Build history of the part. All positions in model axes, mm. Face numbers are marked on the shaded views. A direction names the side the tool comes from. Coordinates: 2 decimals unless noted, no trailing zeros. Write each loop counter-clockwise with the first axis right and the second up, starting at its lowest first coordinate (ties: lowest second). Pieces come first, ordered by that corner, then holes. Notation, with made-up numbers: M 40.25,83.25 L 50.25,83.25 A18 cw 50.25,115.25 Z; hole C -3.75,75.5 d8. An arc over 180 degrees is marked long. Use CSV: the item, a comma, the result in double quotes. Start each with the question number.
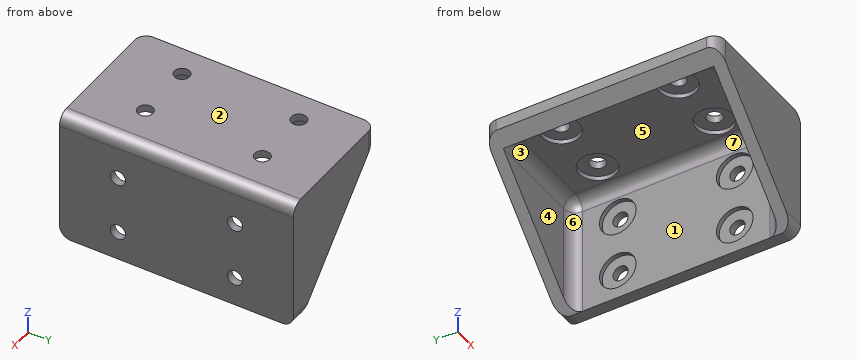
```python
from build123d import *

# Parameters (mm, degrees)
SKETCH1_W           = 45
SKETCH1_H           = 80
BOSS_EXTRUDE1_DEPTH = 45
SKETCH3_R           = 2.6
CUT_EXTRUDE1_DEPTH  = 40
SHELL1_OUTLINE_R    = 6.6
SHELL1_DEPTH        = 41
SHELL1_2_OUTLINE_R  = 6.6
SHELL1_2_DEPTH      = 1
CUT_EXTRUDE2_DEPTH  = 96.338073399
SKETCH5_W           = 37
SKETCH5_H           = 72
CUT_EXTRUDE3_DEPTH  = 40
SKETCH6_R           = 2.6
CUT_EXTRUDE4_DEPTH  = 40
FILLET1_R           = 4
FILLET2_R           = 4
FILLET3_R           = 4
SKETCH8_R           = 6.25
CUT_EXTRUDE5_DEPTH  = 1.5
SKETCH7_R           = 6.25
CUT_EXTRUDE6_DEPTH  = 1.5


# Read off the part's stored shape, not the designer's step: Shell1
with BuildPart() as part:
    # Sketch1 → Boss-Extrude1 (new body)
    with BuildSketch(Plane.XY):
        with Locations((3.274953722, 5.904112676)):
            Rectangle(SKETCH1_W, SKETCH1_H)
    extrude(amount=BOSS_EXTRUDE1_DEPTH)

    # Sketch3 → Cut-Extrude1 (cut)
    with BuildSketch(Plane(origin=(0, 0, 45), x_dir=(-1, 0, 0), z_dir=(0, 0, 1))):
        with Locations(Location((-10.774953722, -25.904112676, 0), (0, 0, 180))):
            Circle(SKETCH3_R)
        with Locations(Location((-10.774953722, 14.095887324, 0), (0, 0, 180))):
            Circle(SKETCH3_R)
        with Locations(Location((9.225046278, 14.095887324, 0), (0, 0, 180))):
            Circle(SKETCH3_R)
        with Locations(Location((9.225046278, -25.904112676, 0), (0, 0, 180))):
            Circle(SKETCH3_R)
    extrude(amount=-CUT_EXTRUDE1_DEPTH, mode=Mode.SUBTRACT)

    # Shell1 outline → Shell1 (cut)
    with BuildSketch(Plane.XY):
        with BuildLine():
            Line((-15.225046278, -16.845432741), (-15.225046278, -30.095887324))
            Line((-15.225046278, -30.095887324), (21.774953722, -30.095887324))
            Line((21.774953722, -30.095887324), (21.774953722, 41.904112676))
            Line((21.774953722, 41.904112676), (-15.225046278, 41.904112676))
            Line((-15.225046278, 41.904112676), (-15.225046278, 28.653658093))
            ThreePointArc((-15.225046278, 28.653658093), (-2.625046278, 25.904112676), (-15.225046278, 23.154567259))
            Line((-15.225046278, 23.154567259), (-15.225046278, -11.346341907))
            ThreePointArc((-15.225046278, -11.346341907), (-2.625046278, -14.095887324), (-15.225046278, -16.845432741))
        make_face()
        with Locations((10.774953722, -14.095887324)):
            Circle(SHELL1_OUTLINE_R, mode=Mode.SUBTRACT)
        with Locations((10.774953722, 25.904112676)):
            Circle(SHELL1_OUTLINE_R, mode=Mode.SUBTRACT)
    extrude(amount=SHELL1_DEPTH, mode=Mode.SUBTRACT)

    # Shell1 2 outline → Shell1 2 (cut)
    with BuildSketch(Plane.XY):
        with BuildLine():
            Line((-15.225046278, -11.346341907), (-15.225046278, -16.845432741))
            ThreePointArc((-15.225046278, -16.845432741), (-2.625046278, -14.095887324), (-15.225046278, -11.346341907))
        make_face()
        with BuildLine():
            Line((-15.225046278, 28.653658093), (-15.225046278, 23.154567259))
            ThreePointArc((-15.225046278, 23.154567259), (-2.625046278, 25.904112676), (-15.225046278, 28.653658093))
        make_face()
        with Locations((10.774953722, -14.095887324)):
            Circle(SHELL1_2_OUTLINE_R)
        with Locations((10.774953722, 25.904112676)):
            Circle(SHELL1_2_OUTLINE_R)
    extrude(amount=SHELL1_2_DEPTH, mode=Mode.SUBTRACT)

    # Sketch4 → Cut-Extrude2 (cut, through all)
    with BuildSketch(Plane(origin=(0, 45.904112676, 0), x_dir=(1, 0, 0), z_dir=(0, 1, 0))):
        Polygon((-19.225046278, 0), (-19.225046278, -41), (21.774953722, 0), align=None)
    extrude(amount=-CUT_EXTRUDE2_DEPTH, mode=Mode.SUBTRACT)

    # Sketch5 → Cut-Extrude3 (cut)
    with BuildSketch(Plane(origin=(0, 0, 41), x_dir=(-1, 0, 0), z_dir=(0, 0, -1))):
        with Locations((-3.274953722, 5.904112676)):
            Rectangle(SKETCH5_W, SKETCH5_H)
    extrude(amount=CUT_EXTRUDE3_DEPTH, mode=Mode.SUBTRACT)

    # Sketch6 → Cut-Extrude4 (cut)
    with BuildSketch(Plane(origin=(25.774953722, 0, 0), x_dir=(0, 0, 1), z_dir=(1, 0, 0))):
        with Locations(Location((10, -25.904112676, 0), (0, 0, 180))):
            Circle(SKETCH6_R)
        with Locations(Location((10, 14.095887324, 0), (0, 0, 180))):
            Circle(SKETCH6_R)
        with Locations(Location((30, 14.095887324, 0), (0, 0, 180))):
            Circle(SKETCH6_R)
        with Locations(Location((30, -25.904112676, 0), (0, 0, 180))):
            Circle(SKETCH6_R)
    extrude(amount=-CUT_EXTRUDE4_DEPTH, mode=Mode.SUBTRACT)

    # Fillet1
    fillet1_edges = [part.edges().sort_by_distance(p)[0] for p in [
        (3.274953722, -30.095887324, 41),
        (21.774953722, -30.095887324, 20.5),
        (21.774953722, 41.904112676, 20.5),
        (21.774953722, 5.904112676, 41),
        (3.274953722, 41.904112676, 41),
    ]]
    fillet(fillet1_edges, radius=FILLET1_R)

    # Fillet2
    fillet2_edges = [part.edges().sort_by_distance(p)[0] for p in [
        (23.774953722, -34.095887324, 0),
        (23.774953722, 45.904112676, 0),
        (-19.225046278, -34.095887324, 43),
        (-19.225046278, 45.904112676, 43),
    ]]
    fillet(fillet2_edges, radius=FILLET2_R)

    # Fillet3
    fillet3_edges = [part.edges().sort_by_distance(p)[0] for p in [
        (25.774953722, 5.904112676, 45),
    ]]
    fillet(fillet3_edges, radius=FILLET3_R)

    # Sketch8 → Cut-Extrude5 (cut)
    with BuildSketch(Plane(origin=(0, 0, 41), x_dir=(-1, 0, 0), z_dir=(0, 0, -1))):
        with Locations((-10.774953722, -14.095887324)):
            Circle(SKETCH8_R)
        with Locations((-10.774953722, 25.904112676)):
            Circle(SKETCH8_R)
        with Locations((9.225046278, 25.904112676)):
            Circle(SKETCH8_R)
        with Locations((9.225046278, -14.095887324)):
            Circle(SKETCH8_R)
    extrude(amount=-CUT_EXTRUDE5_DEPTH, mode=Mode.SUBTRACT)

    # Sketch7 → Cut-Extrude6 (cut)
    with BuildSketch(Plane.ZY.offset(-21.774953722)):
        with Locations((10, 25.904112676)):
            Circle(SKETCH7_R)
        with Locations((30, 25.904112676)):
            Circle(SKETCH7_R)
        with Locations((30, -14.095887324)):
            Circle(SKETCH7_R)
        with Locations((10, -14.095887324)):
            Circle(SKETCH7_R)
    extrude(amount=-CUT_EXTRUDE6_DEPTH, mode=Mode.SUBTRACT)


solid = part.part
```
1. 3-axis set-ups, long thin cutter, end or side, ignore diameter. For the marked faces 1, 2 and 3: which of +Z, -Z, +X, -X, +Y, -Y reach the whole face in a straight line?
2. Pull direction X, two halves, no side cores. Call the marked faces 4, 5, 6 and 7: pulls with the +X half, pulls with the -X half, needs draft (parallel to the pull), parting line crosses it, or undercut.
3. Slice it at B-B (y = 9). List the corners of the cut face in (x, z).
4. Slice it at D-D (z = 10). List the corners of the cut face in (x, y), and give its area (3 significant figures).
5. Drill centre lines: line 1 along Y through (x, z) = (22, 30); line 2 along Y through (x, z) = (5, 42); line 3 along Y through (x, z) = (18, 35.5). Where is each one in solid material? Low to high. Write a range as from..to.
6. Slice it at C-C (x = 1). List the corners of the cut face in (y, z), and give its area (3 significant figures).
7. Slice it at A-A (z = 30). List the corners of the cut face in (x, y), and give its area (3 significant figures).
8. Flat gauge pins, fed straight in: pin 1 (6 mm diameter, centred on y = -11.5, z = 7.5, fed in from -X); pin 2 (4 mm diameter, centred on y = 29.5, z = 37, fed in from -X); pin 3 (7 mm diameter, centred on x = 10.77, y = 25.9, fed in from -Z). Where does each tip first touch, or does it go through?
Established:
1,face 1,"-Z, -X"
1,face 2,"+Z, +X, -X, +Y, -Y"
1,face 3,"-Z"
2,face 4,"needs draft"
2,face 5,"undercut"
2,face 6,"pulls with the -X half"
2,face 7,"undercut"
3,outline,"M -19.23,41 L -15.23,37 L -15.23,41 L 17.77,41 A4 cw 21.77,37 L 21.77,0 L 25.77,0 L 25.77,41 A4 ccw 21.77,45 L -19.23,45 Z"
4,outline,"M 11.77,-34.1 L 25.77,-34.1 L 25.77,-16.7 L 23.27,-16.7 L 23.27,-20.35 L 21.77,-20.35 L 21.77,-26.1 A4 cw 17.77,-30.1 L 11.77,-30.1 Z; M 11.77,41.9 L 17.77,41.9 A4 cw 21.77,37.9 L 21.77,32.15 L 23.27,32.15 L 23.27,28.5 L 25.77,28.5 L 25.77,45.9 L 11.77,45.9 Z; M 21.77,-7.85 L 23.27,-7.85 L 23.27,-11.5 L 25.77,-11.5 L 25.77,23.3 L 23.27,23.3 L 23.27,19.65 L 21.77,19.65 Z"
4,area,"343 mm2"
5,line 1,"y = -34.1..-20.35, -7.85..19.65, 32.15..45.9"
5,line 2,"y = -34.1..-16.49, -11.71..23.51, 28.29..45.9"
5,line 3,"y = -34.1..-30.09, 41.9..45.9"
6,outline,"M -34.1,20.77 L -30.1,20.77 L -30.1,37 A4 cw -26.1,41 L 37.9,41 A4 cw 41.9,37 L 41.9,20.77 L 45.9,20.77 L 45.9,45 L -34.1,45 Z"
6,area,"489 mm2"
7,outline,"M -8.23,-34.1 L 25.77,-34.1 L 25.77,-16.7 L 23.27,-16.7 L 23.27,-20.35 L 21.77,-20.35 L 21.77,-26.1 A4 cw 17.77,-30.1 L -8.23,-30.1 Z; M -8.23,41.9 L 17.77,41.9 A4 cw 21.77,37.9 L 21.77,32.15 L 23.27,32.15 L 23.27,28.5 L 25.77,28.5 L 25.77,45.9 L -8.23,45.9 Z; M 21.77,-7.85 L 23.27,-7.85 L 23.27,-11.5 L 25.77,-11.5 L 25.77,23.3 L 23.27,23.3 L 23.27,19.65 L 21.77,19.65 Z"
7,area,"503 mm2"
8,pin 1,"stops at x = 21.77"
8,pin 2,"stops at x = -17.23"
8,pin 3,"stops at z = 42.5"
